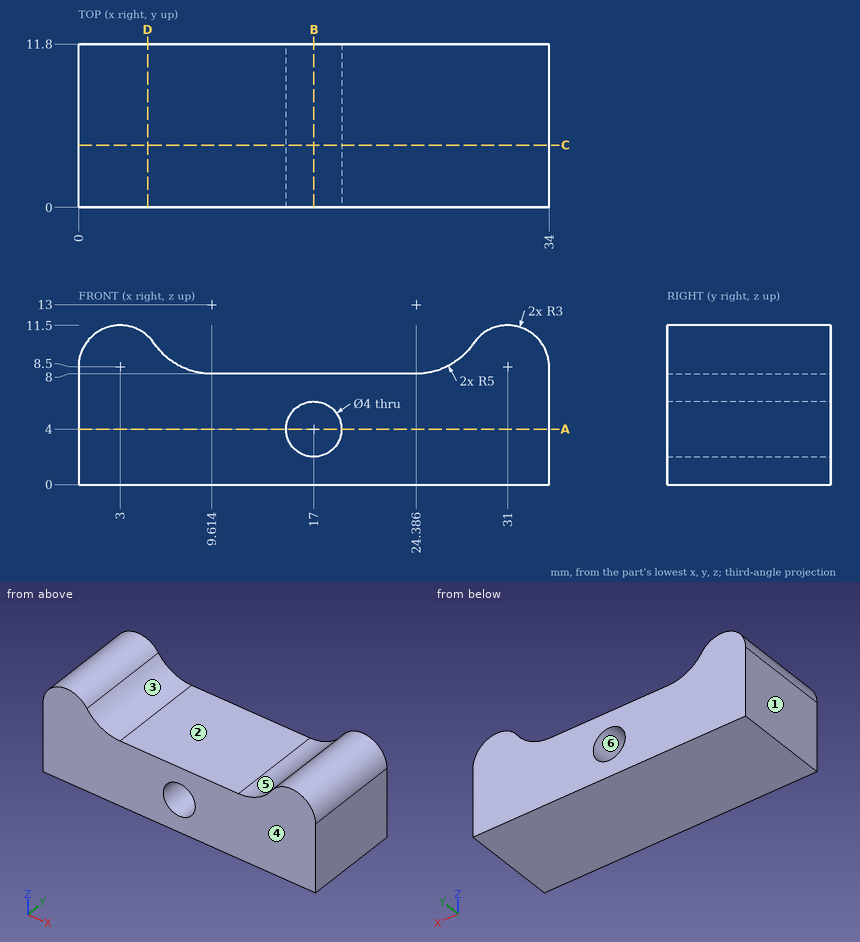
Can you work these out from the drawing? Everything is in mm from the part's minimum corner. A direction names the side the tool comes from. Round coordinates to 2 decimals unless told otherwise and drop trailing zeros. Write each loop counter-clockwise with the first axis right and the second up, starting at its lowest first coordinate (ties: lowest second). Pieces come first, ordered by that corner, then holes.
1. If we mould it in two halves opening along X, with no side actions, what happens to the marked faces 1, 2, 3 and 4? For each: released by +X, released by -X, zero draft, split by the parting line, or undercut.
2. Suppose I cut it at D-D (x = 5). List the corners of the cut face in (y, z) for me.
3. Will these pins go through, and if not, where does the flat tip stop? pin 1 Ø6 at (x, y) = (22.5, 8) entering from +Z; pin 2 Ø1.5 at (x, y) = (8.5, 2.5) entering from +Z; pin 3 Ø3.5 at (x, y) = (14, 4) entering from +Z.
4. I need wall thicknesses on L1, parallel to X at y = 8, z = 4; L2, parallel to Z at x = 17, y = 9; L3, parallel to Z at x = 24, y = 10. Which ranges of each line are inside material? Lowest first, please.
5. For the marked faces 5 and 6, which set-ups out of +Z, -Z, +X, -X, +Y, -Y let a thin tool reach every point of the face, with its end or its side?
6. Suppose I cut it at A-A (z = 4). List the corners of the cut face in (x, y) for me, and give its area (3 significant figures).
7. Suppose I cut it at B-B (x = 17). List the corners of the cut face in (y, z) for me.
8. Suppose I cut it at C-C (y = 4.5). List the corners of the cut face in (x, z) for me (1 decimal), and give its area (3 significant figures).
Answer sheet:
1. face 1: released by -X
1. face 2: undercut
1. face 3: undercut
1. face 4: zero draft
2. outline: (0, 0) - (11.8, 0) - (11.8, 10.74) - (0, 10.74) - close
3. pin 1: stops at z = 8.13
3. pin 2: stops at z = 8.36
3. pin 3: stops at z = 8
4. L1: x = 0 to 15, 19 to 34
4. L2: z = 0 to 2, 6 to 8
4. L3: z = 0 to 8
5. face 5: +Z, +Y, -Y
5. face 6: +Y, -Y
6. outline: (0, 0) - (15, 0) - (15, 11.8) - (0, 11.8) - close; (19, 0) - (34, 0) - (34, 11.8) - (19, 11.8) - close
6. area: 354 mm2
7. outline: (0, 0) - (11.8, 0) - (11.8, 2) - (0, 2) - close; (0, 6) - (11.8, 6) - (11.8, 8) - (0, 8) - close
8. outline: (0, 0) - (34, 0) - (34, 8.5) arc R3 ccw to (28.5, 10.2) arc R5 cw to (24.4, 8) - (9.6, 8) arc R5 cw to (5.5, 10.2) arc R3 ccw to (0, 8.5) - close; hole circle Ø4 at (17, 4)
8. area: 297 mm2
